Input: part model. Units: mm. Frame: model coordinates. A direction names the side the tool comes from. Give positions to 0.01 mm unless a question says otherwise; leave off trailing zeros. Loops run counter-clockwise (first coordinate to the right, second up) from the corner with the lowest first, then second, coordinate; pieces in that order, holes last. Notation, with made-up numbers: (43, -36) - (101, -36) arc R12 ccw to (101, -16) - close; hole circle Ø4 at (-21.75, 87.5). An arc over 180 degrees is marked (long way). Answer as a JSON object with one key per item and string values.
from build123d import *

# Parameters (mm, degrees)
F1_DEPTH = 63.5
F2_DEPTH = 25.4


with BuildPart() as f1:
    # F0 (on Front) → F1 (new body, symmetric)
    with BuildSketch(Plane.XZ):
        Polygon((22.225, 9.525), (-41.275, 9.525), (-41.275, -9.525), (41.275, -9.525), (41.275, 9.525), align=None)
    extrude(amount=F1_DEPTH, both=True)

    # F0 (on Front) → F2 (join, symmetric)
    with BuildSketch(Plane.XZ):
        with BuildLine():
            add(Edge.make_bspline(
                [(-41.275, 9.525), (-7.472832, 31.815227), (2.111726, 70.312925), (60.131503, 76.395682)],
                knots=[0, 0, 0, 0, 121.470025, 121.470025, 121.470025, 121.470025], degree=3))
            Line((-41.275, 9.525), (22.225, 9.525))
            Line((22.225, 9.525), (22.225, 40.7162))
            ThreePointArc((22.225, 40.7162), (32.454296, 65.411904), (57.15, 75.6412))
            Line((57.15, 75.6412), (60.131503, 75.6412))
            Line((60.131503, 75.6412), (60.131503, 76.395682))
        make_face()
        with BuildLine():
            Line((22.225, 40.7162), (22.225, 9.525))
            Line((22.225, 9.525), (41.275, 9.525))
            Line((41.275, 9.525), (41.275, 40.7162))
            ThreePointArc((41.275, 40.7162), (45.92468, 51.94152), (57.15, 56.5912))
            Line((57.15, 56.5912), (60.131503, 56.5912))
            Line((60.131503, 56.5912), (60.131503, 75.6412))
            Line((60.131503, 75.6412), (57.15, 75.6412))
            ThreePointArc((57.15, 75.6412), (32.454296, 65.411904), (22.225, 40.7162))
        make_face()
    extrude(amount=F2_DEPTH, both=True)

    # F0 (on Front) → F3 (revolve)
    with BuildSketch(Plane.XZ):
        Polygon((110.931503, 76.395682), (60.131503, 76.395682), (60.131503, 75.6412), (60.131503, 56.5912), (60.131503, 47.820682), (110.931503, 47.820682), align=None)
    revolve(axis=Axis((60.131503, 0, 62.108182), (0, 0, 1)))


solid = f1.part
Item 1: Cut plane D-D (x = 83). Return loops of the section in (y, z).
Geometry check:
{"outline": "(-45.36, 47.82) - (45.36, 47.82) - (45.36, 76.4) - (-45.36, 76.4) - close"}
Item 2: Access query for faces 5 (the face through (108.586, 15.259, 62.308)), 6 (the face through (-1, 63.5, 0)). Directions: +Z, -Z, +X, -X, +Y, -Y. A direction counts if a zero-diameter tool reaches every point of the face in a straight line with its end or side. Return the directions, or none.
Geometry check:
{"face 5": "+Z", "face 6": "+Z, -Z, +X, -X, +Y"}
Item 3: Cut plane B-B (z = -2). Return loops of the section in (x, y) (3 decimals).
Geometry check:
{"outline": "(-41.275, -63.5) - (41.275, -63.5) - (41.275, 63.5) - (-41.275, 63.5) - close"}
Item 4: Cut plane C-C (y = -39). Return loops of the section in (x, z) (3 decimals), then the cut area to 3 significant figures.
Geometry check:
{"outline": "(-41.275, -9.525) - (41.275, -9.525) - (41.275, 9.525) - (-41.275, 9.525) - close; (27.579, 47.821) - (92.684, 47.821) - (92.684, 76.396) - (27.579, 76.396) - close", "area": "3,430 mm2"}
Item 5: Mould query, pull axis Z, two halves, no side actions, for faces 1 (the face through (41.275, -1, 10)), 2 (the face through (59, 1, 76.396)), 3 (the face through (-1, -1, -9.525)), 4 (the face through (11, 25.4, 30)). Classes: released by +Z, released by -Z, zero draft, split by the parting line, or undercut.
Geometry check:
{"face 1": "zero draft", "face 2": "released by +Z", "face 3": "released by -Z", "face 4": "undercut"}
Item 6: Cut plane A-A (y = 32.5). Return loops of the section in (x, z) (3 decimals).
Geometry check:
{"outline": "(-41.275, -9.525) - (41.275, -9.525) - (41.275, 9.525) - (-41.275, 9.525) - close; (21.088, 47.821) - (99.175, 47.821) - (99.175, 76.396) - (21.088, 76.396) - close"}
Item 7: Contact query for flat-ended pins moving along their axis: P1, Ø3, axis at y = 3, z = 24, coming from the -X side; P2, Ø6, axis at x = 45, y = 49.5, coming from the -Z side; P3, Ø5, axis at x = 14.5, z = 64, coming from the +Y side. Output: stop coordinate, or through.
Geometry check:
{"P1": "stops at x = -25.32", "P2": "stops at z = 47.82", "P3": "stops at y = 26.84"}
Item 8: Material intervals for line 1 (Z direction, x = 37, y = 26.5) (3 decimals); line 2 (Z direction, x = 75, y = -7.5); line 3 (Z direction, x = 12.5, y = -53.5) (3 decimals), sorted ascending. Write a range as [from, to].
Geometry check:
{"line 1": "z = [-9.525, 9.525], [47.821, 76.396]", "line 2": "z = [47.82, 76.4]", "line 3": "z = [-9.525, 9.525]"}
